Here's how the part is built. I have some questions about the finished solid (model axes, mm). Face numbers are marked on the shaded views. A direction names the side the tool comes from. Give positions to 0.01 mm unless a question says otherwise; leave off trailing zeros. Write each loop counter-clockwise with the first axis right and the second up, starting at its lowest first coordinate (ties: lowest second). Pieces come first, ordered by that corner, then holes. Notation, with made-up numbers: (-18.5, 38.5) -> (30.5, 38.5) arc R20 cw to (30.5, 74.5) -> close; hole circle Ø10 at (46.25, -37.5). An arc over 180 degrees is marked (long way). Return JSON: item names as keys, results as strings.
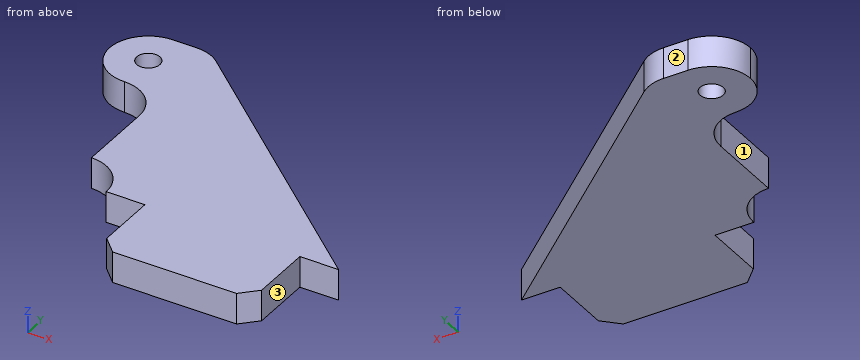
from build123d import *

# Parameters (mm, degrees)
F0_R     = 0.75
F1_DEPTH = 2
F2_R     = 2.49999


# Not quite as in the source:
# - a fillet or chamfer is up to 0.001 mm smaller than in the source, because OpenCascade refuses the exact size


with BuildPart() as f1:
    # F0 (on Top) → F1 (new body)
    with BuildSketch(Plane.XY):
        with BuildLine():
            Line((-10, 0), (-7.5, 0))
            Line((-7.5, 0), (2.5, 0))
            Line((2.5, 0), (5, 0))
            Line((5, 0), (-12.5, 15))
            Line((-12.5, 15), (-17.5, 15))
            Line((-17.5, 15), (-17.5, 10))
            Line((-17.5, 10), (-12.5, 10))
            Line((-12.5, 10), (-12.5, 2.5))
            ThreePointArc((-12.5, 2.5), (-10.732233047, 1.767766953), (-10, 0))
        make_face()
        with Locations((-15, 12.5)):
            Circle(F0_R, mode=Mode.SUBTRACT)
        Polygon((-7.5, -4), (-6.5, -5), (1.5, -5), (2.5, -4), (2.5, 0), (-7.5, 0), align=None)
    extrude(amount=F1_DEPTH)

    # F2 (radius 2.5 in the source; OpenCascade refuses exactly that, so slightly less here)
    f2_edges = [f1.edges().sort_by_distance(p)[0] for p in [
        (-17.5, 15, 1),
        (-17.5, 10, 1),
        (-12.5, 15, 1),
        (-12.5, 10, 1),
    ]]
    fillet(f2_edges, radius=F2_R)


solid = f1.part
1. Suppose I cut it at B-B, the plane y = 12.75. List the corners of the cut face in (x, z) for me (3 decimals), and give its area (3 significant figures).
Taken from the geometry:
{"outline": "(-17.487, 0) -> (-15.707, 0) -> (-15.707, 2) -> (-17.487, 2) -> close; (-14.293, 0) -> (-9.875, 0) -> (-9.875, 2) -> (-14.293, 2) -> close", "area": "12.4 mm²"}
2. Suppose I cut it at D-D, the plane y = 9. List the corners of the cut face in (x, z) for me, and give its area (3 significant figures).
Taken from the geometry:
{"outline": "(-13, 0) -> (-5.5, 0) -> (-5.5, 2) -> (-13, 2) -> close", "area": "15.0 mm²"}
3. Which directions (+Z, -Z, +X, -X, +Y, -Y) give clear straight access to the entire face, cutting with the end or side of a thin tool? Please do the marked faces 1, 2 and 3.
Taken from the geometry:
{"face 1": "+Z, -Z, -X, -Y", "face 2": "+Z, -Z, +X, -X, +Y", "face 3": "+Z, -Z, +X, -Y"}
4. Suppose I cut it at C-C, the plane x = -2. List the corners of the cut face in (y, z) for me, and give its area (3 significant figures).
Taken from the geometry:
{"outline": "(-5, 0) -> (6, 0) -> (6, 2) -> (-5, 2) -> close", "area": "22.0 mm²"}
5. For pin 1 Ø1 at (x, z) = (-8.5, 1) entering from -Y; pin 2 Ø5 at (x, y) = (-4, 12) entering from +Z; pin 3 Ø1 at (y, z) = (9.5, 1) entering from +X; pin 4 Ø0.6 at (y, z) = (-1.5, 1) entering from +X, each with a flat end and sliding along its axis, tell me the tip position at first contact or that it passes through.
Taken from the geometry:
{"pin 1": "stops at y = 0", "pin 2": "passes through", "pin 3": "stops at x = -5.5", "pin 4": "stops at x = 2.5"}
6. If I drill on line 1 (Y direction, x = -15, z = 0.8); line 2 (X direction, y = -3, z = 0.45); line 3 (X direction, y = 8.75, z = 1.2), over which ranges is the centre line in solid material (lowest first)? Write a range as [from, to].
Taken from the geometry:
{"line 1": "y = [10, 11.75], [13.25, 15]", "line 2": "x = [-7.5, 2.5]", "line 3": "x = [-12.83, -5.21]"}
